Geometry: see drawing. Coordinates: mm, zero at the bounding-box minimum. Round coordinates to 2 decimals unless told otherwise and drop trailing zeros. Loops run counter-clockwise (first coordinate to the right, second up) from the corner with the lowest first, then second, coordinate; pieces in that order, holes last.
(1) Section A-A, the plane y = 24.5. Return the cut outline in (x, z).
(2) Material intervals for probe 1 along Y at (x, z) = (25.5, 1.35); probe 2 along Y at (x, z) = (64.5, 1.55); probe 3 along X at (y, z) = (37.5, 1.9), sorted ascending.
(3) First-contact query: pin 1 Ø2 at (x, y) = (25.5, 38.4) entering from +Z. Flat tip, straight axial feed; report the tip coordinate or a pass-through.
(4) Section C-C, the plane x = 70.5. Return the cut outline in (y, z), plus the area to 3 significant figures.
(5) Section B-B, the plane z = 0.55. Return the cut outline in (x, y), plus the area to 3 significant figures.
(6) Section D-D, the plane x = 48. Return the cut outline in (y, z), plus the area to 3 significant figures.
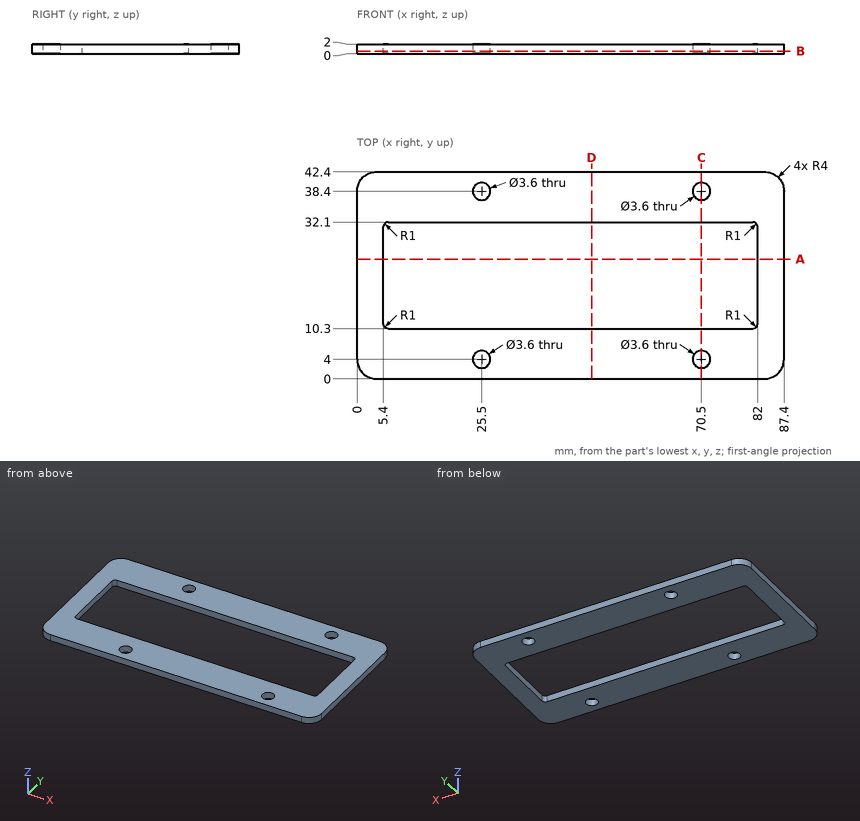
Output values:
1. outline: (0, 0) - (5.4, 0) - (5.4, 2) - (0, 2) - close; (82, 0) - (87.4, 0) - (87.4, 2) - (82, 2) - close
2. probe 1: y = 0 to 2.2, 5.8 to 10.3, 32.1 to 36.6, 40.2 to 42.4
2. probe 2: y = 0 to 10.3, 32.1 to 42.4
2. probe 3: x = 0 to 23.94, 27.06 to 68.94, 72.06 to 87.4
3. pin 1: passes through
4. outline: (0, 0) - (2.2, 0) - (2.2, 2) - (0, 2) - close; (5.8, 0) - (10.3, 0) - (10.3, 2) - (5.8, 2) - close; (32.1, 0) - (36.6, 0) - (36.6, 2) - (32.1, 2) - close; (40.2, 0) - (42.4, 0) - (42.4, 2) - (40.2, 2) - close
4. area: 26.8 mm2
5. outline: (0, 4) arc R4 ccw to (4, 0) - (83.4, 0) arc R4 ccw to (87.4, 4) - (87.4, 38.4) arc R4 ccw to (83.4, 42.4) - (4, 42.4) arc R4 ccw to (0, 38.4) - close; hole (5.4, 11.3) arc R1 ccw to (6.4, 10.3) - (81, 10.3) arc R1 ccw to (82, 11.3) - (82, 31.1) arc R1 ccw to (81, 32.1) - (6.4, 32.1) arc R1 ccw to (5.4, 31.1) - close; hole circle Ø3.6 at (25.5, 4); hole circle Ø3.6 at (25.5, 38.4); hole circle Ø3.6 at (70.5, 4); hole circle Ø3.6 at (70.5, 38.4)
5. area: 1,980 mm2
6. outline: (0, 0) - (10.3, 0) - (10.3, 2) - (0, 2) - close; (32.1, 0) - (42.4, 0) - (42.4, 2) - (32.1, 2) - close
6. area: 41.2 mm2
